The model under review builds one solid part; all positions refer to its coordinate system, in mm. Face numbers are marked on the shaded views. A direction names the side the tool comes from. Round coordinates to 2 decimals unless told otherwise and drop trailing zeros. Write each loop counter-clockwise with the first axis right and the second up, starting at its lowest first coordinate (ties: lowest second). Pieces come first, ordered by that corner, then holes. Notation, with made-up numbers: M 80,46 L 120,46 A17 cw 120,51 Z; hole C 13.25,78 d7. An arc over 180 degrees is marked long. One line per item, written item: value. Start each with the question number.
1) Take a section at C-C, the plane x = 26. Write out the cut boundary in (y, z).
2) For P1, Ø5, axis at y = 5, z = -9, coming from the +X side; P2, Ø12, axis at x = 11, y = 5, coming from the +Z side; P3, Ø1.5, axis at x = 33.5, y = -6, coming from the +Z side; P4, Ø12, axis at y = -9.5, z = -4.5, coming from the -X side, all flat-tipped, find the tip position at first contact; note any pin that passes through.
3) Tool access review of the marked faces 1, 2 and 3: name each direction out of +Z, -Z, +X, -X, +Y, -Y from which nothing blocks a thin tool from reaching the whole face with its end or side.
4) Wall thickness on probe 1 along X at (y, z) = (2, -2.5); probe 2 along Z at (x, y) = (12, -0.25); probe 3 along Z at (x, y) = (14, 1.5): over which ranges is each line inside the solid? List them lowest first.
5) Take a section at A-A, the plane z = 0. Write out the cut boundary in (x, y), and give its area (3 significant figures).
from build123d import *

# Parameters (mm, degrees)
F0_R     = 12.7
F1_DEPTH = 38.1
F2_SIZE  = 1.27
F3_R     = 2.54
F4_DEPTH = 4.064
F5_R     = 2.54
F6_DEPTH = 4.064


with BuildPart() as f1:
    # F0 (on Right) → F1 (new body)
    with BuildSketch(Plane.YZ):
        Circle(F0_R)
    extrude(amount=F1_DEPTH)

    # F2
    f2_edges = [f1.edges().sort_by_distance(p)[0] for p in [
        (0, -12.7, 0),
        (19.05, 12.7, 0),
        (38.1, -12.7, 0),
    ]]
    chamfer(f2_edges, length=F2_SIZE)

    # F3 (on face) → F4 (join)
    with BuildSketch(Plane(origin=(0, 0, 0), x_dir=(0, -1, 0), z_dir=(-1, 0, 0))):
        Circle(F3_R)
    extrude(amount=F4_DEPTH)

    # F5 (on face) → F6 (join)
    with BuildSketch(Plane.YZ.offset(38.1)):
        Circle(F5_R)
    extrude(amount=F6_DEPTH)


solid = f1.part
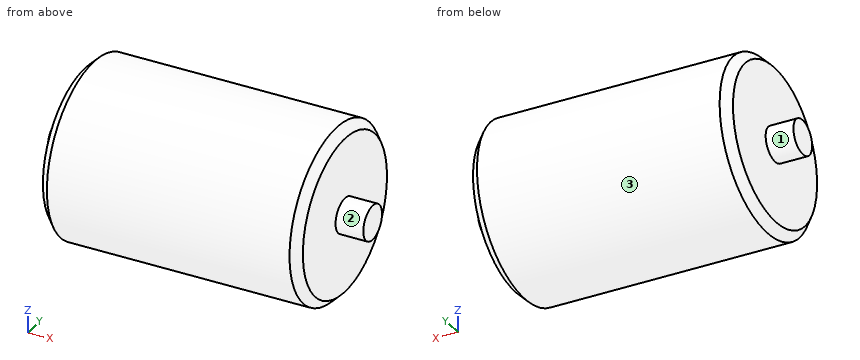
Checked values:
1. outline: C 0,0 d25.4
2. P1: stops at x = 38.1
2. P2: stops at z = 12.7
2. P3: stops at z = 11.56
2. P4: stops at x = 0
3. face 1: -X
3. face 2: +X
3. face 3: +X, -X
4. probe 1: x = 0 to 38.1
4. probe 2: z = -12.7 to 12.7
4. probe 3: z = -12.61 to 12.61
5. outline: M -4.06,-2.54 L 0,-2.54 L 0,-11.43 L 1.27,-12.7 L 36.83,-12.7 L 38.1,-11.43 L 38.1,-2.54 L 42.16,-2.54 L 42.16,2.54 L 38.1,2.54 L 38.1,11.43 L 36.83,12.7 L 1.27,12.7 L 0,11.43 L 0,2.54 L -4.06,2.54 Z
5. area: 1,010 mm2
